from build123d import *

# Parameters (mm, degrees)
SKETCH1_W           = 130
SKETCH1_H           = 430
BOSS_EXTRUDE1_DEPTH = 3
SKETCH2_W           = 30
SKETCH2_H           = 40
CUT_EXTRUDE1_DEPTH  = 10
SKETCH3_R           = 1.5
SKETCH3_R_2         = 2.1
CUT_EXTRUDE2_DEPTH  = 10
SKETCH4_R           = 7
CUT_EXTRUDE3_DEPTH  = 10


with BuildPart() as part:
    # Sketch1 → Boss-Extrude1 (new body)
    with BuildSketch(Plane(origin=(0, 0, 0), x_dir=(1, 0, 0), z_dir=(0, 1, 0))):
        Rectangle(SKETCH1_W, SKETCH1_H)
    extrude(amount=BOSS_EXTRUDE1_DEPTH)

    # Sketch2 → Cut-Extrude1 (cut)
    with BuildSketch(Plane(origin=(0, 3, 0), x_dir=(1, 0, 0), z_dir=(0, 1, 0))):
        with Locations((0, -195)):
            Rectangle(SKETCH2_W, SKETCH2_H)
    extrude(amount=-CUT_EXTRUDE1_DEPTH, mode=Mode.SUBTRACT)

    # Sketch3 → Cut-Extrude2 (cut)
    with BuildSketch(Plane.XZ):
        with Locations(Location((-53.05, -3.75, 0), (0, 0, 270))):
            Circle(SKETCH3_R)
        with Locations(Location((-46.5, 195, 0), (0, 0, 270))):
            Circle(SKETCH3_R)
        with Locations(Location((-24.95, -3.75, 0), (0, 0, 270))):
            Circle(SKETCH3_R)
        with Locations(Location((-53.05, -106.75, 0), (0, 0, 270))):
            Circle(SKETCH3_R)
        with Locations(Location((46.5, 195, 0), (0, 0, 270))):
            Circle(SKETCH3_R)
        with Locations(Location((-24.95, -106.75, 0), (0, 0, 270))):
            Circle(SKETCH3_R)
        with Locations(Location((24.95, -106.75, 0), (0, 0, 90))):
            Circle(SKETCH3_R)
        with Locations(Location((57.5, 202.5, 0), (0, 0, 270))):
            Circle(SKETCH3_R)
        with Locations(Location((53.05, -106.75, 0), (0, 0, 90))):
            Circle(SKETCH3_R)
        with Locations(Location((24.95, -3.75, 0), (0, 0, 90))):
            Circle(SKETCH3_R)
        with Locations(Location((-57.5, 202.5, 0), (0, 0, 270))):
            Circle(SKETCH3_R)
        with Locations(Location((53.05, -3.75, 0), (0, 0, 90))):
            Circle(SKETCH3_R)
        with Locations(Location((-41.5, 175, 0), (0, 0, 270))):
            Circle(SKETCH3_R_2)
        with Locations(Location((41.5, 175, 0), (0, 0, 270))):
            Circle(SKETCH3_R_2)
        with Locations(Location((41.5, -175, 0), (0, 0, 270))):
            Circle(SKETCH3_R_2)
        with Locations(Location((-41.5, -175, 0), (0, 0, 270))):
            Circle(SKETCH3_R_2)
    extrude(amount=-CUT_EXTRUDE2_DEPTH, mode=Mode.SUBTRACT)

    # Sketch4 → Cut-Extrude3 (cut)
    with BuildSketch(Plane.XZ):
        with Locations(Location((-17.5, 100.952208061, 0), (0, 0, 270))):
            Circle(SKETCH4_R)
        with Locations(Location((17.5, 100.952208061, 0), (0, 0, 270))):
            Circle(SKETCH4_R)
    extrude(amount=-CUT_EXTRUDE3_DEPTH, mode=Mode.SUBTRACT)


solid = part.part
Can you work these out from the model? Positions are in its coordinate system, mm. Round coordinates to 2 decimals unless told otherwise and drop trailing zeros. Loops run counter-clockwise (first coordinate to the right, second up) from the corner with the lowest first, then second, coordinate; pieces in that order, holes last. Notation, with made-up numbers: (80, 83) - (123, 83) arc R21 cw to (123, 97) - close; hole circle Ø4 at (-26, 68). An arc over 180 degrees is marked (long way). Use CSV: the item, a comma, the result in double quotes. Start each with the question number.
1) We'd pull the mould along Z, two halves only. Please class faces 1 (the flat face through (-1, 0, -3)), 2 (the cylindrical face through (-20.181, 1.479, 94.486)), 3 (the cylindrical face through (14.819, 1.479, 94.486)): released by +Z, released by -Z, zero draft, split by the parting line, or undercut.
2) If we section it at B-B on x = 3.5: Write out the boundary of the cut face in (y, z), plus the area to 3 significant figures.
3) For pin 1 Ø2.5 at (x, z) = (-24.95, -3.75) entering from +Y; pin 2 Ø1.5 at (x, y) = (7, 1.5) entering from +Z, each with a flat end and sliding along its axis, tell me the tip position at first contact or that it passes through.
4) If we section it at A-A on y = 1.05: Count the separate pieces of the cut face and the enclosed holes in it, plus the area to 3 significant figures.
5) Please list where these lines run through material, in increasing order: probe 1 along X at (y, z) = (1.75, -3.75); probe 2 along Z at (x, y) = (24.95, 1.2); probe 3 along X at (y, z) = (0.9, -175). Write a range as [from, to].
Geometry results:
1,face 1,"zero draft"
1,face 2,"undercut"
1,face 3,"undercut"
2,outline,"(0, -215) - (3, -215) - (3, 175) - (0, 175) - close"
2,area,"1,170 mm2"
3,pin 1,"passes through"
3,pin 2,"stops at z = 175"
4,separate pieces,"1"
4,enclosed holes,"18"
4,area,"54,300 mm2"
5,probe 1,"x = [-65, -54.55], [-51.55, -26.45], [-23.45, 23.45], [26.45, 51.55], [54.55, 65]"
5,probe 2,"z = [-215, -108.25], [-105.25, -5.25], [-2.25, 215]"
5,probe 3,"x = [-65, -43.6], [-39.4, 39.4], [43.6, 65]"
